from build123d import *

# Parameters (mm, degrees)
SKETCH1_W                    = 120
SKETCH1_H                    = 85
BASE_EXTRUSION_DEPTH         = 35
EXTERNAL_CORNER_FILLETS_R    = 3
ENCLOSURE_SHELL_T            = -2.5
SKETCH2_R                    = 4
SKETCH2_R_2                  = 1.5875
ARDUINO_MOUNTING_HOLES_DEPTH = 6
STANDOFF_FILLETS_R           = 1
PORT_ACCESS_HOLE_DEPTH       = 6
SKETCH5_W                    = 15
SKETCH5_H                    = 8
WIRE_ACCESS_HOLE_DEPTH       = 6
WIRE_ACCESS_HOLE_FILLET_R    = 2
SKETCH6_R                    = 2.5
CABLE_ROUTING_POSTS_DEPTH    = 6
LID_CUT_EXTRUDE_DEPTH        = 117.5


with BuildPart() as part:
    # Sketch1 → base extrusion (new body)
    with BuildSketch(Plane(origin=(0, 0, 0), x_dir=(1, 0, 0), z_dir=(0, 1, 0))):
        Rectangle(SKETCH1_W, SKETCH1_H)
    extrude(amount=BASE_EXTRUSION_DEPTH)

    # external corner fillets
    external_corner_fillets_edges = [part.edges().sort_by_distance(p)[0] for p in [
        (60, 17.5, 42.5),
        (60, 17.5, -42.5),
        (-60, 17.5, -42.5),
        (-60, 17.5, 42.5),
    ]]
    fillet(external_corner_fillets_edges, radius=EXTERNAL_CORNER_FILLETS_R)

    # enclosure shell
    enclosure_shell_openings = [part.faces().sort_by_distance(p)[0] for p in [
        (0, 35, 0),
    ]]
    offset(amount=ENCLOSURE_SHELL_T, openings=enclosure_shell_openings, kind=Kind.INTERSECTION)

    # Sketch2 → arduino mounting holes (add)
    # profile 1 of 4: a face of its own
    with BuildSketch(Plane.XZ):
        with Locations(Location((-37.18, 29.719377118, 0), (0, 0, 270))):
            Circle(SKETCH2_R)
        with Locations(Location((-37.18, 29.719377118, 0), (0, 0, 270))):
            Circle(SKETCH2_R_2, mode=Mode.SUBTRACT)
    # profile 2 of 4: a face of its own
    with BuildSketch(Plane.XZ):
        with Locations(Location((14.89, 24.639377118, 0), (0, 0, 270))):
            Circle(SKETCH2_R)
        with Locations(Location((14.89, 24.639377118, 0), (0, 0, 270))):
            Circle(SKETCH2_R_2, mode=Mode.SUBTRACT)
    # profile 3 of 4: a face of its own
    with BuildSketch(Plane.XZ):
        with Locations(Location((14.89, -3.300622882, 0), (0, 0, 270))):
            Circle(SKETCH2_R)
        with Locations(Location((14.89, -3.300622882, 0), (0, 0, 270))):
            Circle(SKETCH2_R_2, mode=Mode.SUBTRACT)
    # profile 4 of 4: a face of its own
    with BuildSketch(Plane.XZ):
        with Locations(Location((-35.91, -18.540622882, 0), (0, 0, 270))):
            Circle(SKETCH2_R)
        with Locations(Location((-35.91, -18.540622882, 0), (0, 0, 270))):
            Circle(SKETCH2_R_2, mode=Mode.SUBTRACT)
    extrude(amount=-ARDUINO_MOUNTING_HOLES_DEPTH)

    # standoff fillets
    standoff_fillets_edges = [part.edges().sort_by_distance(p)[0] for p in [
        (-35.91, 2.5, -14.540622882),
        (14.89, 2.5, 0.699377118),
        (14.89, 2.5, 28.639377118),
        (-37.18, 2.5, 33.719377118),
    ]]
    fillet(standoff_fillets_edges, radius=STANDOFF_FILLETS_R)

    # Sketch4 → port access hole (cut)
    with BuildSketch(Plane.ZY.offset(60)):
        with BuildLine():
            Line((20.584377118, 18.65), (28.584377118, 18.65))
            ThreePointArc((28.584377118, 18.65), (28.937930508, 18.503553391), (29.084377118, 18.15))
            Line((29.084377118, 18.15), (29.084377118, 7.65))
            Line((29.084377118, 7.65), (20.084377118, 7.65))
            Line((20.084377118, 7.65), (20.084377118, 18.15))
            ThreePointArc((20.084377118, 18.15), (20.230823727, 18.503553391), (20.584377118, 18.65))
        make_face()
        with BuildLine():
            Line((-11.320622882, 18.7), (-0.200622882, 18.7))
            ThreePointArc((-0.200622882, 18.7), (0.124646237, 18.565269119), (0.259377118, 18.24))
            Line((0.259377118, 18.24), (0.259377118, 8.44))
            ThreePointArc((0.259377118, 8.44), (0.122186575, 8.182772563), (-0.150622882, 8.08))
            Line((-0.150622882, 8.08), (-11.370622882, 8.08))
            ThreePointArc((-11.370622882, 8.08), (-11.660536663, 8.20008622), (-11.780622882, 8.49))
            Line((-11.780622882, 8.49), (-11.780622882, 18.24))
            ThreePointArc((-11.780622882, 18.24), (-11.645892002, 18.565269119), (-11.320622882, 18.7))
        make_face()
    extrude(amount=-PORT_ACCESS_HOLE_DEPTH, mode=Mode.SUBTRACT)

    # Sketch5 → wire access hole (cut)
    with BuildSketch(Plane(origin=(60, 0, 0), x_dir=(0, 0, -1), z_dir=(1, 0, 0))):
        with Locations((27, 10)):
            Rectangle(SKETCH5_W, SKETCH5_H)
    extrude(amount=-WIRE_ACCESS_HOLE_DEPTH, mode=Mode.SUBTRACT)

    # wire access hole fillet
    wire_access_hole_fillet_edges = [part.edges().sort_by_distance(p)[0] for p in [
        (58.75, 14, -34.5),
        (58.75, 6, -34.5),
        (58.75, 6, -19.5),
        (58.75, 14, -19.5),
    ]]
    fillet(wire_access_hole_fillet_edges, radius=WIRE_ACCESS_HOLE_FILLET_R)

    # Sketch6 → cable routing posts (add)
    with BuildSketch(Plane(origin=(0, 2.5, 0), x_dir=(1, 0, 0), z_dir=(0, 1, 0))):
        with Locations(Location((40.747327805, 27, 0), (0, 0, 90))):
            Circle(SKETCH6_R)
        with Locations(Location((40.747327805, 15.750588276, 0), (0, 0, 90))):
            Circle(SKETCH6_R)
    extrude(amount=CABLE_ROUTING_POSTS_DEPTH)

    # Sketch10 → lid cut extrude (cut)
    with BuildSketch(Plane.ZY.offset(60)):
        Polygon((-39.5, 35), (-39.5, 32.6), (-41, 32.6), (-41, 30.8), (41, 30.8), (41, 32.6), (39.5, 32.6), (39.5, 35), align=None)
    extrude(amount=-LID_CUT_EXTRUDE_DEPTH, mode=Mode.SUBTRACT)


solid = part.part
Can you work these out from the model? Positions are in its coordinate system, mm. A direction names the side the tool comes from. Give positions to 0.01 mm unless a question says otherwise; leave off trailing zeros. Write each loop counter-clockwise with the first axis right and the second up, starting at its lowest first coordinate (ties: lowest second). Pieces come first, ordered by that corner, then holes. Notation, with made-up numbers: M 75,-15 L 90,-15 A20 ccw 90,23 Z; hole C 74.5,16 d11. An arc over 180 degrees is marked long. Answer in a Markdown table with one row per item. Add a question column.
Item 1: Imagine slicing it at C-C, the plane x = -13.5. Write out the boundary of the cut face in (y, z), plus the area to 3 significant figures.
Item 2: We'd pull the mould along X, two halves only. Please class faces 1 (the flat face through (59, 6, -27)), 2 (the cylindrical face through (59.1, 17.74, 41.64)), 3 (the flat face through (-1, 34, -40)): released by +X, released by -X, zero draft, split by the parting line, or undercut.
Item 3: Imagine slicing it at A-A, the plane y = 29.5. Write out the boundary of the cut face in (x, z).
Item 4: For pin 1 Ø1 at (x, z) = (14.5, -3.5) entering from +Y; pin 2 Ø2.5 at (x, z) = (-36.5, 31.5) entering from +Y; pin 3 Ø2 at (x, z) = (-59.5, -3.5) entering from +Y, each with a flat end and sliding along its axis, tell me the tip position at first contact or that it passes through.
Item 5: Please list where these lines run through material, in increasing order: L1, parallel to Z at x = 26.5, y = 13; L2, parallel to X at y = 13.5, z = -16.5; L3, parallel to Y at x = -18, z = 23.
Item 6: On a 3-axis mill with a long thin cutter (end or side, diameter ignored), from which of +Z, -Z, +X, -X, +Y, -Y can I reach the whole of each face in a straight line? I mean faces 4 (the flat face through (59, 14, -27)), 5 (the flat face through (-59, 13, -11.781)), 6 (the flat face through (-59, 34, 39.5)), 7 (the cylindrical face through (15.96, 4.23, 25.81)). Say none if no direction works.
Item 7: Imagine slicing it at D-D, the plane z = -27. Write out the boundary of the cut face in (x, y).
Item 8: Imagine slicing it at B-B, the plane z = 18. Write out the boundary of the cut face in (x, y).
Evaluation:
| question | item | result |
|---|---|---|
| 1 | outline | M 0,-42.5 L 35,-42.5 L 35,-40 L 32.6,-40 L 32.6,-41 L 30.8,-41 L 30.8,-40 L 2.5,-40 L 2.5,40 L 30.8,40 L 30.8,41 L 32.6,41 L 32.6,40 L 35,40 L 35,42.5 L 0,42.5 Z |
| 1 | area | 371 mm² |
| 2 | face 1 | zero draft |
| 2 | face 2 | released by +X |
| 2 | face 3 | undercut |
| 3 | outline | M -60,-39.5 A3 ccw -57,-42.5 L 57,-42.5 A3 ccw 60,-39.5 L 60,39.5 A3 ccw 57,42.5 L -57,42.5 A3 ccw -60,39.5 Z; hole M -57.5,-39.5 A0.5 ccw -57,-40 L 57,-40 A0.5 ccw 57.5,-39.5 L 57.5,39.5 A0.5 ccw 57,40 L -57,40 A0.5 ccw -57.5,39.5 Z |
| 4 | pin 1 | stops at y = 2.5 |
| 4 | pin 2 | stops at y = 6 |
| 4 | pin 3 | stops at y = 30.8 |
| 5 | L1 | z = -42.5 to -40, 40 to 42.5 |
| 5 | L2 | x = -60 to -57.5, 57.5 to 60 |
| 5 | L3 | y = 0 to 2.5 |
| 6 | face 4 | +X |
| 6 | face 5 | -X |
| 6 | face 6 | -X, +Y |
| 6 | face 7 | +Y |
| 7 | outline | M -60,0 L 60,0 L 60,6 L 57.5,6 L 57.5,2.5 L 43.25,2.5 L 43.25,8.5 L 38.25,8.5 L 38.25,2.5 L -57.5,2.5 L -57.5,30.8 L -60,30.8 Z; M 57.5,14 L 60,14 L 60,35 L 57.5,35 Z |
| 8 | outline | M -60,0 L 60,0 L 60,35 L 57.5,35 L 57.5,2.5 L -57.5,2.5 L -57.5,30.8 L -60,30.8 Z |
